The listing builds one solid part. Answer for the finished solid, in the listing's coordinates (mm). Give positions to 0.01 mm unless a question says otherwise; leave off trailing zeros. Loops run counter-clockwise (first coordinate to the right, second up) from the corner with the lowest first, then second, coordinate; pieces in that order, holes last. Notation, with made-up numbers: (18, 39.5) -> (60, 39.5) arc R37 ccw to (60, 76.5) -> close; hole circle Ø3 at (-4, 28.25). An arc over 180 degrees is marked (long way). One line per question, with ' | ' between items. Start each with the question number.
from build123d import *

# Parameters (mm, degrees)
BASE_FLANGE1_DEPTH = 10
SKETCH6_R          = 6.75
SKETCH6_R_2        = 10
CUT_EXTRUDE1_DEPTH = 496.075751779
FILLET1_R          = 10


# Sheet-metal steps are written as plain solids
with BuildPart() as part:
    # Sketch1 → Base-Flange1 (new body)
    with BuildSketch(Plane.XY):
        with BuildLine():
            Line((-350, 190), (-350, 270))
            ThreePointArc((-350, 270), (-326.568542495, 326.568542495), (-270, 350))
            Line((-270, 350), (-190, 350))
            Line((-190, 350), (-190, 230))
            Line((-190, 230), (-230, 190))
            Line((-230, 190), (-350, 190))
        make_face()
    extrude(amount=BASE_FLANGE1_DEPTH)

    # Sketch6 → Cut-Extrude1 (cut, through all)
    with BuildSketch(Plane(origin=(0, 0, 0), x_dir=(-1, 0, 0), z_dir=(0, 0, -1))):
        with Locations((270, 310)):
            Circle(SKETCH6_R)
        with Locations((310, 270)):
            Circle(SKETCH6_R)
        with Locations((230, 270)):
            Circle(SKETCH6_R)
        with Locations((270, 230)):
            Circle(SKETCH6_R)
        with Locations((270, 270)):
            Circle(SKETCH6_R_2)
    extrude(amount=-CUT_EXTRUDE1_DEPTH, mode=Mode.SUBTRACT)

    # Fillet1
    fillet1_edges = [part.edges().sort_by_distance(p)[0] for p in [
        (-190, 350, 5),
        (-190, 230, 5),
        (-230, 190, 5),
        (-350, 190, 5),
    ]]
    fillet(fillet1_edges, radius=FILLET1_R)


solid = part.part
1. Determine the mould class of faces 1 (the flat face through (-190, 288, 5)), 2 (the cylindrical face through (-327.19, 325.94, 4.93)), 3 (the cylindrical face through (-274.614, 261.128, 4.93)) for opening direction Y: released by +Y, released by -Y, zero draft, split by the parting line, or undercut.
2. The part is cut by section C-C (x = -266). Write down the section's boundary in (y, z), plus the area to 3 significant figures.
3. The part is cut by section D-D (x = -310). Write down the section's boundary in (y, z), plus the area to 3 significant figures.
4. The part is cut by section B-B (y = 230). Write down the section's boundary in (x, z).
5. Each of these flat-tipped pins is pushed along its axis until it touches: pin 1 Ø1 at (y, z) = (331, 9) entering from -X; pin 2 Ø12 at (x, y) = (-310, 270) entering from +Z (3 decimals); pin 3 Ø1 at (y, z) = (324, 6) entering from -X. Where does it stop, or does it pass through?
6. The part is cut by section A-A (z = 3.75). Write down the section's boundary in (x, y).
7. Straight lines are drawn through the part: L1, parallel to Y at x = -270, z = 7.5; L2, parallel to Y at x = -272, z = 5.5 (3 decimals); L3, parallel to Y at x = -310, z = 5. For each, find the intervals that lie inside material, in ascending order.
Check sheet entries:
1) face 1: zero draft | face 2: released by +Y | face 3: undercut
2) outline: (190, 0) -> (224.56, 0) -> (224.56, 10) -> (190, 10) -> close; (235.44, 0) -> (260.83, 0) -> (260.83, 10) -> (235.44, 10) -> close; (279.17, 0) -> (304.56, 0) -> (304.56, 10) -> (279.17, 10) -> close; (315.44, 0) -> (350, 0) -> (350, 10) -> (315.44, 10) -> close | area: 1,200 mm^2
3) outline: (190, 0) -> (263.25, 0) -> (263.25, 10) -> (190, 10) -> close; (276.75, 0) -> (339.28, 0) -> (339.28, 10) -> (276.75, 10) -> close | area: 1,360 mm^2
4) outline: (-350, 0) -> (-276.75, 0) -> (-276.75, 10) -> (-350, 10) -> close; (-263.25, 0) -> (-190.9, 0) -> (-190.9, 10) -> (-263.25, 10) -> close
5) pin 1: stops at x = -322.34 | pin 2: passes through | pin 3: stops at x = -329.48
6) outline: (-350, 200) arc R10 ccw to (-340, 190) -> (-234.14, 190) arc R10 ccw to (-227.07, 192.93) -> (-192.93, 227.07) arc R10 ccw to (-190, 234.14) -> (-190, 340) arc R10 ccw to (-200, 350) -> (-270, 350) arc R80 ccw to (-350, 270) -> close; hole circle Ø13.5 at (-310, 270); hole circle Ø20 at (-270, 270); hole circle Ø13.5 at (-270, 230); hole circle Ø13.5 at (-270, 310); hole circle Ø13.5 at (-230, 270)
7) L1: y = 190 to 223.25, 236.75 to 260, 280 to 303.25, 316.75 to 350 | L2: y = 190 to 223.553, 236.447 to 260.202, 279.798 to 303.553, 316.447 to 349.975 | L3: y = 190 to 263.25, 276.75 to 339.28
